Source: CAD feature listing. Evaluate the final solid. Frame: model axes, mm. A direction names the side the tool comes from. Round coordinates to 2 decimals unless told otherwise and drop trailing zeros. Write each loop counter-clockwise with the first axis right and the second up, starting at its lowest first coordinate (ties: lowest second). Pieces come first, ordered by that corner, then holes. Notation, with made-up numbers: M 84,36.5 L 118,36.5 A22 ccw 118,53.5 Z; hole C 39,6 d1. An arc over 180 degrees is marked long. Use a Markdown table: item, result.
Autodesk Inventor part; units mm, degrees
ref_plane "YZ Plane" through (0, 0, 0) normal (1, 0, 0) x (0, 1, 0)
ref_plane "XZ Plane" through (0, 0, 0) normal (0, 1, 0) x (-1, 0, 0)
ref_plane "XY Plane" through (0, 0, 0) normal (0, 0, 1) x (1, 0, 0)
sketch "Sketch1" plane through (0, 0, 0) normal (0, 0, 1) x (1, 0, 0)
  line L0 (25.4, -110.3376) -> (-25.4, -110.3376)
  line L1 (-25.4, -110.3376) -> (-25.4, 110.3376)
  line L2 (-25.4, 110.3376) -> (25.4, 110.3376)
  line L3 (25.4, 110.3376) -> (25.4, -110.3376)
  line L4 (25.4, -110.3376) -> (-25.4, 110.3376) construction
  line L5 (-25.4, -110.3376) -> (25.4, 110.3376) construction
  line L6 (25.4, 110.3376) -> (152.8069, -110.3376)
  line L7 (25.4, 110.3376) -> (280.2138, 110.3376) construction
  line L8 (152.8069, -110.3376) -> (25.4, -110.3376)
  point P0 (0, 0)
  dimension "d0" = 50.8
  dimension "d1" = 220.6752
  dimension "d2" = 60
extrude "Extrusion1" add sketch "Sketch1" along normal blind 3.175
sketch "Sketch2" plane through (0, 0, 3.175) normal (0, 0, 1) x (1, 0, 0)
  line L0 (152.8069, -110.3376) -> (25.4, 110.3376)
  line L1 (-25.4, -110.3376) -> (152.8069, -110.3376)
  line L2 (152.8069, -107.1626) -> (-25.4, -107.1626)
  line L3 (-25.4, -107.1626) -> (-25.4, -110.3376)
  line L4 (150.9738, -107.1626) -> (152.8069, -110.3376)
  point P0 (0, 0)
  dimension "d5" = 3.175
extrude "Extrusion2" add sketch "Sketch2" along normal blind 12.7
sketch "Sketch3" plane through (0, 0, 3.175) normal (0, 0, 1) x (1, 0, 0)
  line L0 (-25.4, 110.3376) -> (0, 110.3376)
  line L1 (0, 110.3376) -> (0, 84.9376)
  line L2 (0, 84.9376) -> (-25.4, 84.9376)
  line L3 (-25.4, 84.9376) -> (-25.4, 110.3376)
  circle A0 centre (0, 84.9376) radius 14.2875
  point P0 (0, 0)
  dimension "d8" = 25.4
  dimension "d9" = 25.4
  dimension "d10" = 28.575
extrude "Extrusion3" cut sketch "Sketch3" against normal blind 25.4 contours A0 L2 L1 | L1 L2 A0
properties part number "LPlate"
Q1. Section D-D on x = 89.5. Return loops of the section in (y, z) (3 decimals), plus the area to 3 significant figures.
Results are:
| item | result |
|---|---|
| outline | M -110.338,0 L -0.687,0 L -0.687,3.175 L -107.163,3.175 L -107.163,15.875 L -110.338,15.875 Z |
| area | 388 mm^2 |
Q2. Section A-A on x = 0. Return loops of the section in (y, z) (3 decimals), plus the area to 3 significant figures.
Results are:
| item | result |
|---|---|
| outline | M -110.338,0 L 70.65,0 L 70.65,3.175 L -107.163,3.175 L -107.163,15.875 L -110.338,15.875 Z; M 99.225,0 L 110.338,0 L 110.338,3.175 L 99.225,3.175 Z |
| area | 650 mm^2 |
Q3. Reachability of faces 1 (the flat face through (43, -23, 0)), 2 (the flat face through (42, -21, 3.175)) from +Z, -Z, +X, -X, +Y, -Y: full face, straight path, thin tool, end or side. Return the list, or none.
Results are:
| item | result |
|---|---|
| face 1 | -Z, +X, -X, +Y, -Y |
| face 2 | +Z, +X, -X, +Y |
Q4. Mould query, pull axis Y, two halves, no side actions, for faces 3 (the flat face through (89.4, -0.51, 1.43)), 4 (the cylindrical face through (-3.1, 70.99, 1.61)), 5 (the flat face through (-25.4, 1, 1)). Classes: +Y half, -Y half, draft (parallel to the pull), parting line (faces both ways), or undercut.
Results are:
| item | result |
|---|---|
| face 3 | +Y half |
| face 4 | undercut |
| face 5 | draft |
Q5. First-contact query: pin 1 Ø1.5 at (x, y) = (5, -45.5) entering from +Z (3 decimals); pin 2 Ø1.5 at (x, z) = (32, 3) entering from +Y. Flat tips, straight axial feed; report the tip coordinate or a pass-through.
Results are:
| item | result |
|---|---|
| pin 1 | z = 3.175 |
| pin 2 | y = 100.21 |
Q6. Section B-B on z = 12.75. Return loops of the section in (x, y), plus the area to 3 significant figures.
Results are:
| item | result |
|---|---|
| outline | M -25.4,-110.34 L 152.81,-110.34 L 150.97,-107.16 L -25.4,-107.16 Z |
| area | 563 mm^2 |
Q7. Line query: L1, parallel to Y at x = 0, z = 1.65; L2, parallel to Z at x = 68, y = -2 (3 decimals); L3, parallel to Y at x = 51, z = 5.25. Output: solid intervals per line, ascending.
Results are:
| item | result |
|---|---|
| L1 | -110.34 to 70.65, 99.23 to 110.34 |
| L2 | 0 to 3.175 |
| L3 | -110.34 to -107.16 |
Q8. Section C-C on y = 19.5. Return loops of the section in (x, z) (3 decimals), plus the area to 3 significant figures.
Results are:
| item | result |
|---|---|
| outline | M -25.4,0 L 77.845,0 L 77.845,3.175 L -25.4,3.175 Z |
| area | 328 mm^2 |
